from build123d import *

# Parameters (mm, degrees)
SCHIZZO1_R                   = 21.5
ESTRUSIONE_ESTRUSIONE1_DEPTH = 20
SCHIZZO2_R                   = 4
TAGLIO_ESTRUSIONE1_DEPTH     = 20


with BuildPart() as part:
    # Schizzo1 → Estrusione-Estrusione1 (new body)
    with BuildSketch(Plane.XY):
        Polygon((0, 0), (95, 0), (95, 61), (81, 75), (14, 75), (0, 61), align=None)
        with Locations((47.5, 40)):
            Circle(SCHIZZO1_R, mode=Mode.SUBTRACT)
    extrude(amount=ESTRUSIONE_ESTRUSIONE1_DEPTH)

    # Schizzo2 → Taglio-Estrusione1 (cut)
    with BuildSketch(Plane.XZ):
        with Locations(Location((47.5, 10, 0), (0, 0, 270))):
            Circle(SCHIZZO2_R)
        with Locations(Location((17.5, 10, 0), (0, 0, 270))):
            Circle(SCHIZZO2_R)
        with Locations(Location((77.5, 10, 0), (0, 0, 90))):
            Circle(SCHIZZO2_R)
    extrude(amount=-TAGLIO_ESTRUSIONE1_DEPTH, mode=Mode.SUBTRACT)


solid = part.part
Read the model definition and answer for the solid it produces. Units are mm, in the model's axes. A direction names the side the tool comes from. Round coordinates to 2 decimals unless told otherwise and drop trailing zeros. Order: outer loops, then holes, each group sorted by start corner. A loop starts at its lowest first (then second) coordinate and runs counter-clockwise, first axis right, second up.
1) For faces 1 (the face through (18, 20, 10)), 2 (the face through (47, 0, 5)), determine the directions among +Z, -Z, +X, -X, +Y, -Y from which every point of the face is accessible in a straight line to the end or side of a thin tool.
2) The part is cut by section B-B on y = 40. Write down the section's boundary in (x, z).
3) The mould has two halves that part along Z. Classify faces 3 (the face through (95, 30, 10)), 4 (the face through (21.466, 9.86, 10.521)), 5 (the face through (45.1, 9.3, 13.2)), 6 (the face through (36, 21, 20)): released by +Z, released by -Z, zero draft, split by the parting line, or undercut.
4) Flat-ended cylindrical pins translate along their axes: pin 1 (9 mm diameter, centred on x = 79, z = 10.5, fed in from -Y); pin 2 (2.5 mm diameter, centred on x = 18.5, z = 11.5, fed in from -Y). Find the tip coordinate at first contact, or state that the pin passes through.
5) The part is cut by section A-A on x = 47.5. Write down the section's boundary in (y, z), plus the area to 3 significant figures.
6) The part is cut by section C-C on z = 2.75. Write down the section's boundary in (x, y).
7) Straight lines are drawn through the part: L1, parallel to X at y = 13.25, z = 10; L2, parallel to Z at x = 77.5, y = 8.25; L3, parallel to Y at x = 35, z = 12.75. For each, find the intervals that lie inside material, in ascending order.
8) The part is cut by section D-D on x = 77.5. Write down the section's boundary in (y, z), plus the area to 3 significant figures.
Resolved:
1. face 1: -Y
1. face 2: +Z, -Z, +X, -X, -Y
2. outline: (0, 0) - (26, 0) - (26, 20) - (0, 20) - close; (69, 0) - (95, 0) - (95, 20) - (69, 20) - close
3. face 3: zero draft
3. face 4: undercut
3. face 5: undercut
3. face 6: released by +Z
4. pin 1: stops at y = 0
4. pin 2: stops at y = 20
5. outline: (0, 0) - (18.5, 0) - (18.5, 6) - (0, 6) - close; (0, 14) - (18.5, 14) - (18.5, 20) - (0, 20) - close; (61.5, 0) - (75, 0) - (75, 20) - (61.5, 20) - close
5. area: 492 mm2
6. outline: (0, 0) - (95, 0) - (95, 61) - (81, 75) - (14, 75) - (0, 61) - close; hole circle Ø43 at (47.5, 40)
7. L1: x = 0 to 13.5, 21.5 to 43.5, 51.5 to 73.5, 81.5 to 95
7. L2: z = 0 to 6, 14 to 20
7. L3: y = 0 to 22.51, 57.49 to 75
8. outline: (0, 0) - (75, 0) - (75, 20) - (0, 20) - (0, 14) - (20, 14) - (20, 6) - (0, 6) - close
8. area: 1,340 mm2
